Read the model definition and answer for the solid it produces. Units are mm, in the model's axes. Give positions to 0.01 mm unless a question says otherwise; leave off trailing zeros. Order: outer loops, then holes, each group sorted by start corner. A loop starts at its lowest first (then second) coordinate and runs counter-clockwise, first axis right, second up.
Item 1: Given pin 1 Ø1.5 at (y, z) = (7, 8) entering from -X; pin 2 Ø1.2 at (x, z) = (92, 4) entering from -Y; pin 3 Ø2 at (y, z) = (12.5, 4) entering from +X, each flat-ended and moving along its own axis, determine where each tip first touches the part or whether it passes through.
Item 2: A cutting plane is placed at C-C (y = -2). Write down the section's boundary in (x, z) (3 decimals).
Item 3: A cutting plane is placed at B-B (x = 132). Write down the section's boundary in (y, z), plus the area to 3 significant figures.
Item 4: A cutting plane is placed at A-A (y = -51). Write down the section's boundary in (x, z) (1 decimal).
Item 5: Find the intervals of material crossed by line 1 along X through (y, z) = (-34, 3.25); line 2 along Z through (x, y) = (59.5, -44); line 3 along X through (y, z) = (-49, 4.5), in increasing order.
Item 6: A cutting plane is placed at D-D (y = 19.5). Write down the section's boundary in (x, z) (3 decimals).
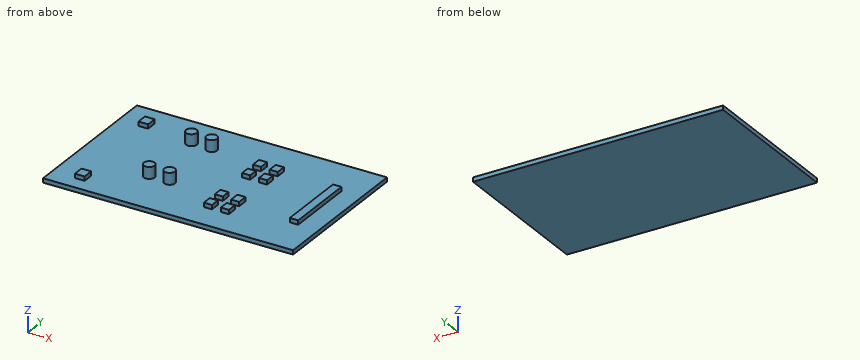
Autodesk Inventor part; units mm, degrees
ref_plane "YZ Plane" through (0, 0, 0) normal (1, 0, 0) x (0, 1, 0)
ref_plane "XZ Plane" through (0, 0, 0) normal (0, 1, 0) x (-1, 0, 0)
ref_plane "XY Plane" through (0, 0, 0) normal (0, 0, 1) x (1, 0, 0)
sketch "Sketch1" plane through (0, 0, 0) normal (0, 0, 1) x (1, 0, 0)
  line L0 (151.1214, 28.1918) -> (4.845, 28.1918)
  line L1 (4.845, 28.1918) -> (4.845, -61.9764)
  line L2 (4.845, -61.9764) -> (151.1214, -61.9764)
  line L3 (151.1214, -61.9764) -> (151.1214, 28.1918)
  point P0 (0, 0)
extrude "Extrusion1" add sketch "Sketch1" along normal blind 2.5
sketch "Sketch2" plane through (0, 0, 2.5) normal (0, 0, 1) x (1, 0, 0)
  line L0 (16.8135, 16.3028) -> (22.4756, 16.3028)
  line L1 (22.4756, 16.3028) -> (22.4756, 10.0115)
  line L2 (22.4756, 10.0115) -> (16.8135, 10.0115)
  line L3 (16.8135, 10.0115) -> (16.8135, 16.3028)
  line L4 (18.3863, -47.2391) -> (24.0485, -47.2391)
  line L5 (24.0485, -47.2391) -> (24.0485, -53.5303)
  line L6 (24.0485, -53.5303) -> (18.3863, -53.5303)
  line L7 (18.3863, -53.5303) -> (18.3863, -47.2391)
  line L8 (89.3205, 6.7086) -> (94.0389, 6.7086)
  line L9 (94.0389, 6.7086) -> (94.0389, 0.8892)
  line L10 (94.0389, 0.8892) -> (89.3205, 0.8892)
  line L11 (89.3205, 0.8892) -> (89.3205, 6.7086)
  line L12 (99.2282, 6.5498) -> (103.9467, 6.5498)
  line L13 (103.9467, 6.5498) -> (103.9467, 0.7304)
  line L14 (103.9467, 0.7304) -> (99.2282, 0.7304)
  line L15 (99.2282, 0.7304) -> (99.2282, 6.5498)
  line L16 (89.3205, -4.037) -> (94.0389, -4.037)
  line L17 (94.0389, -4.037) -> (94.0389, -9.4978)
  line L18 (94.0389, -9.4978) -> (89.3205, -9.4978)
  line L19 (89.3205, -9.4978) -> (89.3205, -4.037)
  line L20 (99.2282, -4.037) -> (103.9467, -4.037)
  line L21 (103.9467, -4.037) -> (103.9467, -9.5401)
  line L22 (103.9467, -9.5401) -> (99.2282, -9.5401)
  line L23 (99.2282, -9.5401) -> (99.2282, -4.037)
  line L24 (134.3826, 3.7989) -> (139.3028, 3.7989)
  line L25 (139.3028, 3.7989) -> (139.3028, -37.6548)
  line L26 (139.3028, -37.6548) -> (134.3826, -37.6548)
  line L27 (134.3826, -37.6548) -> (134.3826, 3.7989)
  line L28 (89.3205, -30.3157) -> (94.0389, -30.3157)
  line L29 (94.0389, -30.3157) -> (94.0389, -35.7312)
  line L30 (94.0389, -35.7312) -> (89.3205, -35.7312)
  line L31 (89.3205, -35.7312) -> (89.3205, -30.3157)
  line L32 (99.2282, -30.3157) -> (103.9467, -30.3157)
  line L33 (103.9467, -30.3157) -> (103.9467, -36.3609)
  line L34 (103.9467, -36.3609) -> (99.2282, -36.3609)
  line L35 (99.2282, -36.3609) -> (99.2282, -30.3157)
  line L36 (99.2282, -40.517) -> (103.9467, -40.517)
  line L37 (103.9467, -40.517) -> (103.9467, -46.1844)
  line L38 (103.9467, -46.1844) -> (99.2282, -46.1844)
  line L39 (99.2282, -46.1844) -> (99.2282, -40.517)
  line L40 (89.3205, -40.517) -> (94.0614, -40.517)
  line L41 (94.0614, -40.517) -> (94.0614, -46.1844)
  line L42 (94.0614, -46.1844) -> (89.3205, -46.1844)
  line L43 (89.3205, -46.1844) -> (89.3205, -40.517)
  point P0 (0, 0)
extrude "Extrusion2" add sketch "Sketch2" along normal blind 2.5
sketch "Sketch3" plane through (0, 0, 2.5) normal (0, 0, 1) x (1, 0, 0)
  circle A0 centre (48.9712, 8.1491) radius 3.1363
  circle A1 centre (60.8345, 8.1491) radius 3.1363
  circle A2 centre (48.9712, -32.3541) radius 3.1454
  circle A3 centre (60.8345, -32.3541) radius 3.1363
  point P0 (0, 0)
extrude "Extrusion3" add sketch "Sketch3" along normal blind 6.75
properties part number "pcb"
Response values:
1. pin 1: stops at x = 45.86
1. pin 2: stops at y = -46.18
1. pin 3: stops at x = 22.48
2. outline: (4.845, 0) - (151.121, 0) - (151.121, 2.5) - (139.303, 2.5) - (139.303, 5) - (134.383, 5) - (134.383, 2.5) - (4.845, 2.5) - close
3. outline: (-61.98, 0) - (28.19, 0) - (28.19, 2.5) - (-61.98, 2.5) - close
3. area: 225 mm2
4. outline: (4.8, 0) - (151.1, 0) - (151.1, 2.5) - (24, 2.5) - (24, 5) - (18.4, 5) - (18.4, 2.5) - (4.8, 2.5) - close
5. line 1: x = 46.29 to 51.65, 58.16 to 63.5, 89.32 to 94.04, 99.23 to 103.95, 134.38 to 139.3
5. line 2: z = 0 to 2.5
5. line 3: x = 18.39 to 24.05
6. outline: (4.845, 0) - (151.121, 0) - (151.121, 2.5) - (4.845, 2.5) - close
